```python
from build123d import *

# Parameters (mm, degrees)
SKETCH_1_W                         = 105
SKETCH_1_H                         = 25
SM_BASE_FLANGE_1_DEPTH             = 1.6
SM_EDGE_FLANGE_1_STRIP_W           = 7.8732
SM_EDGE_FLANGE_1_STRIP_H           = 1.6
SM_EDGE_FLANGE_1_STRIP_CUT_DEPTH   = 105
SM_EDGE_FLANGE_1_STRIP_2_W         = 7.8732
SM_EDGE_FLANGE_1_STRIP_2_H         = 1.6
SM_EDGE_FLANGE_1_STRIP_CUT_2_DEPTH = 105
SM_EDGE_FLANGE_1_DEPTH             = 105
SM_EDGE_FLANGE_1_BEND_DEPTH        = 105
CUT_EXTRUDE_1_DEPTH                = 56.779117956
CUT_EXTRUDE_1_DEPTH_BACK           = 56.779117956
SKETCH_13_R                        = 2
CUT_EXTRUDE_2_DEPTH                = 56.442492729


# Sheet-metal steps are written as plain solids
with BuildPart() as part:
    # Sketch 1 → 基体-法兰1 (new body)
    with BuildSketch(Plane.XY):
        Rectangle(SKETCH_1_W, SKETCH_1_H)
    extrude(amount=-SM_BASE_FLANGE_1_DEPTH)

    # 边线-法兰1 strip (across the edge) → 边线-法兰1 strip cut (cut)
    with BuildSketch(Plane(origin=(-52.5, 12.5, -1.6), x_dir=(0, -1, 0), z_dir=(1, 0, 0))):
        with Locations((-3.2, -0.8)):
            Rectangle(SM_EDGE_FLANGE_1_STRIP_W, SM_EDGE_FLANGE_1_STRIP_H)
    extrude(amount=SM_EDGE_FLANGE_1_STRIP_CUT_DEPTH, mode=Mode.SUBTRACT)

    # 边线-法兰1 strip 2 (across the edge) → 边线-法兰1 strip cut 2 (cut)
    with BuildSketch(Plane(origin=(52.5, -12.5, -1.6), x_dir=(0, 1, 0), z_dir=(-1, 0, 0))):
        with Locations((-3.2, -0.8)):
            Rectangle(SM_EDGE_FLANGE_1_STRIP_2_W, SM_EDGE_FLANGE_1_STRIP_2_H)
    extrude(amount=SM_EDGE_FLANGE_1_STRIP_CUT_2_DEPTH, mode=Mode.SUBTRACT)

    # 边线-法兰1 section (across the edge) → 边线-法兰1 (add)
    with BuildSketch(Plane(origin=(-52.5, 12.5, -1.6), x_dir=(0, -1, 0), z_dir=(1, 0, 0))):
        with BuildLine():
            Line((-1.6, 0.7366), (-1.6, 10.9))
            Line((-1.6, 10.9), (0, 10.9))
            Line((0, 10.9), (0, 0.7366))
            ThreePointArc((0, 0.7366), (0.215745145, 0.215745145), (0.7366, 0))
            Line((0.7366, 0), (0.7366, -1.6))
            ThreePointArc((0.7366, -1.6), (-0.915625705, -0.915625705), (-1.6, 0.7366))
        make_face()
    extrude(amount=SM_EDGE_FLANGE_1_DEPTH)

    # 边线-法兰1 section 2 (across the edge) → 边线-法兰1 bend (add)
    with BuildSketch(Plane(origin=(52.5, -12.5, -1.6), x_dir=(0, 1, 0), z_dir=(-1, 0, 0))):
        with BuildLine():
            Line((-1.6, 0.7366), (-1.6, 10.9))
            Line((-1.6, 10.9), (0, 10.9))
            Line((0, 10.9), (0, 0.7366))
            ThreePointArc((0, 0.7366), (0.215745145, 0.215745145), (0.7366, 0))
            Line((0.7366, 0), (0.7366, -1.6))
            ThreePointArc((0.7366, -1.6), (-0.915625705, -0.915625705), (-1.6, 0.7366))
        make_face()
    extrude(amount=SM_EDGE_FLANGE_1_BEND_DEPTH)

    # 草图12 → 切除-拉伸1 (cut, two sides: drawn at the far end of the back side and taken through both)
    with BuildSketch(Plane(origin=(0, 0, 0), x_dir=(1, 0, 0), z_dir=(0, 1, 0)).offset(-CUT_EXTRUDE_1_DEPTH_BACK)):
        Polygon((-52.5, 8.5), (-48.5, 12.5), (-52.5, 12.5), align=None)
        Polygon((48.5, 12.5), (52.5, 12.5), (52.5, 8.5), align=None)
    extrude(amount=CUT_EXTRUDE_1_DEPTH + CUT_EXTRUDE_1_DEPTH_BACK, mode=Mode.SUBTRACT)

    # 草图13 → 切除-拉伸2 (cut, through all)
    with BuildSketch(Plane(origin=(0, 0, -1.6), x_dir=(-1, 0, 0), z_dir=(0, 0, -1))):
        with Locations((-37.5, 0)):
            Circle(SKETCH_13_R)
    cut_extrude_2 = extrude(amount=-CUT_EXTRUDE_2_DEPTH, mode=Mode.SUBTRACT)

    # 镜向1: 切除-拉伸2 across plane
    add(cut_extrude_2.mirror(Plane(origin=(0, 0, 0), x_dir=(0, 0, 1), z_dir=(1, 0, 0))), mode=Mode.SUBTRACT)


solid = part.part
```
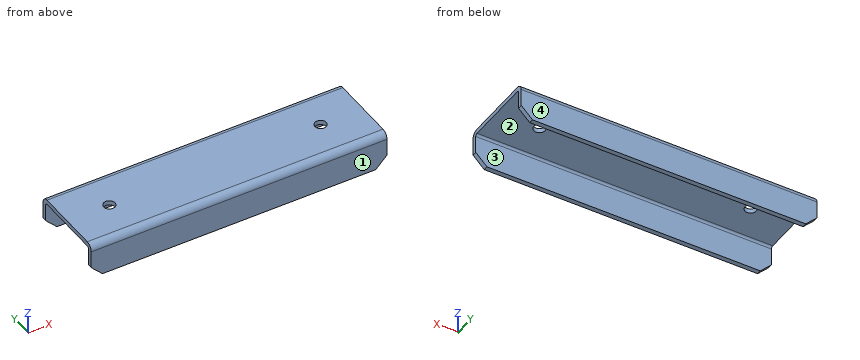
For this review, take the finished solid that the model builds, in its own axes (mm). Face numbers are marked on the shaded views. Coordinates: 2 decimals unless noted, no trailing zeros. Write each loop counter-clockwise with the first axis right and the second up, starting at its lowest first coordinate (ties: lowest second). Pieces come first, ordered by that corner, then holes. Notation, with made-up numbers: (-34.75, 64.25) -> (-0.75, 64.25) arc R20 cw to (-0.75, 84.25) -> close; hole circle Ø8 at (79.5, -32). An arc over 180 degrees is marked (long way). Put each result on its own line as item: value.
Q1. Take a section at B-B, the plane z = -4. State the section outline as (x, y) points.
From the geometry:
outline: (-52.5, -14.1) -> (52.5, -14.1) -> (52.5, -12.5) -> (-52.5, -12.5) -> close; (-52.5, 12.5) -> (52.5, 12.5) -> (52.5, 14.1) -> (-52.5, 14.1) -> close
Q2. The part is to be moulded in two halves that separate along Y. For the marked faces 1, 2, 3 and 4, say which applies: +Y half, -Y half, draft (parallel to the pull), parting line (faces both ways), or undercut.
From the geometry:
face 1: -Y half
face 2: undercut
face 3: undercut
face 4: +Y half
Q3. Take a section at D-D, the plane x = 14. State the section outline as (y, z) points, then the cut area to 3 significant figures.
From the geometry:
outline: (-14.1, -12.5) -> (-12.5, -12.5) -> (-12.5, -2.34) arc R0.74 cw to (-11.76, -1.6) -> (11.76, -1.6) arc R0.74 cw to (12.5, -2.34) -> (12.5, -12.5) -> (14.1, -12.5) -> (14.1, -2.34) arc R2.34 ccw to (11.76, 0) -> (-11.76, 0) arc R2.34 ccw to (-14.1, -2.34) -> close
area: 77.9 mm2
Q4. Take a section at A-A, the plane x = 37.5. State the section outline as (y, z) points, then the cut area to 3 significant figures.
From the geometry:
outline: (-14.1, -12.5) -> (-12.5, -12.5) -> (-12.5, -2.34) arc R0.74 cw to (-11.76, -1.6) -> (-2, -1.6) -> (-2, 0) -> (-11.76, 0) arc R2.34 ccw to (-14.1, -2.34) -> close; (2, -1.6) -> (11.76, -1.6) arc R0.74 cw to (12.5, -2.34) -> (12.5, -12.5) -> (14.1, -12.5) -> (14.1, -2.34) arc R2.34 ccw to (11.76, 0) -> (2, 0) -> close
area: 71.5 mm2
Q5. Clearance check with a flat-ended pin moving along its axis: pin 1 Ø6 at (x, y) = (37, -1.5) entering from -Z. State where the tip first meets the part, or that it passes through.
From the geometry:
pin 1: stops at z = -1.6
Q6. Wall thickness on L1, parallel to Y at x = -42.5, z = -7.25; L2, parallel to Z at x = -14.5, y = -7; L3, parallel to Y at x = 37.5, z = -0.75: over which ranges is each line inside the solid? List them lowest first.
From the geometry:
L1: y = -14.1 to -12.5, 12.5 to 14.1
L2: z = -1.6 to 0
L3: y = -13.48 to -2, 2 to 13.48
Q7. Take a section at C-C, the plane y = 0. State the section outline as (x, z) points.
From the geometry:
outline: (-52.5, -1.6) -> (-39.5, -1.6) -> (-39.5, 0) -> (-52.5, 0) -> close; (-35.5, -1.6) -> (35.5, -1.6) -> (35.5, 0) -> (-35.5, 0) -> close; (39.5, -1.6) -> (52.5, -1.6) -> (52.5, 0) -> (39.5, 0) -> close
